The listing builds one solid part. Answer for the finished solid, in the listing's coordinates (mm). Round coordinates to 2 decimals unless told otherwise and drop trailing zeros. Loops run counter-clockwise (first coordinate to the right, second up) from the corner with the lowest first, then second, coordinate; pieces in that order, holes last. Notation, with made-up numbers: (-26.75, -37) -> (10.25, -37) arc R29 ccw to (10.25, -10) -> close; hole circle Ø7 at (72, 58). An arc over 180 degrees is marked (long way). Answer in a Markdown table with one row per item. Add a question column.
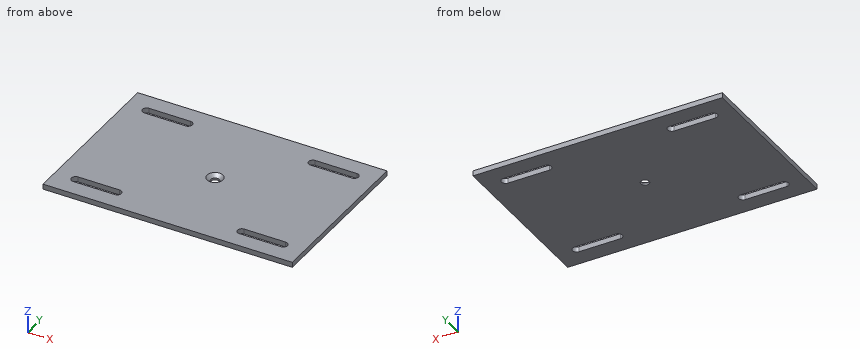
```python
from build123d import *

# Parameters (mm, degrees)
SKETCH1_W            = 152.4
SKETCH1_H            = 101.6
BOSS_EXTRUDE1_DEPTH  = 3.175
CUT_EXTRUDE1_DEPTH   = 92.636022529
MIRROR2_COPY_1_DEPTH = 92.636022529


with BuildPart() as part:
    # Sketch1 → Boss-Extrude1 (new body)
    with BuildSketch(Plane.XY):
        Rectangle(SKETCH1_W, SKETCH1_H)
    extrude(amount=BOSS_EXTRUDE1_DEPTH)

    # Sketch2 → Cut-Extrude1 (cut, symmetric)
    with BuildSketch(Plane.XY.offset(3.175)):
        with BuildLine():
            Line((-63.5, 40.665937046), (-38.1, 40.665937046))
            ThreePointArc((-38.1, 40.665937046), (-35.534062954, 38.1), (-38.1, 35.534062954))
            Line((-38.1, 35.534062954), (-63.5, 35.534062954))
            ThreePointArc((-63.5, 35.534062954), (-66.065937046, 38.1), (-63.5, 40.665937046))
        make_face()
    cut_extrude1 = extrude(amount=CUT_EXTRUDE1_DEPTH, both=True, mode=Mode.SUBTRACT)

    # Mirror1: Cut-Extrude1 across plane
    add(cut_extrude1.mirror(Plane(origin=(0, 0, 0), x_dir=(0, 0, 1), z_dir=(1, 0, 0))), mode=Mode.SUBTRACT)

    # Mirror2: Cut-Extrude1 across plane
    add(cut_extrude1.mirror(Plane.ZX), mode=Mode.SUBTRACT)

    # Mirror2 copy 1 sketch → Mirror2 copy 1 (cut, symmetric)
    with BuildSketch(Plane(origin=(0, 0, 3.175), x_dir=(-1, 0, 0), z_dir=(0, 0, 1))):
        with BuildLine():
            Line((-63.5, 40.665937046), (-38.1, 40.665937046))
            ThreePointArc((-38.1, 40.665937046), (-35.534062954, 38.1), (-38.1, 35.534062954))
            Line((-38.1, 35.534062954), (-63.5, 35.534062954))
            ThreePointArc((-63.5, 35.534062954), (-66.065937046, 38.1), (-63.5, 40.665937046))
        make_face()
    extrude(amount=MIRROR2_COPY_1_DEPTH, both=True, mode=Mode.SUBTRACT)

    # Sketch5 → CSK for #10 Flat Head Machine Screw (100)1 (revolve, cut)
    with BuildSketch(Plane(origin=(0, 0, 3.175), x_dir=(0, -1, 0), z_dir=(1, 0, 0))):
        Polygon((0, 0), (0, 3.175), (2.5527, 3.175), (2.5527, 1.960808018), (4.8895, 0), align=None)
    revolve(axis=Axis((0, 0, 9.525), (0, 0, -1)), mode=Mode.SUBTRACT)


solid = part.part
```
Item 1: Section C-C, the plane z = 0.5 is taken. Write down the section's boundary in (x, y).
Item 2: Flat-ended cylindrical pins translate along their axes: P1, Ø4, axis at x = 0, y = 0, coming from the +Z side; P2, Ø5, axis at x = 0, y = 27, coming from the -Z side. Find the tip coordinate at first contact, or state that the pin passes through.
Item 3: Section B-B, the plane y = 38.1 is taken. Write down the section's boundary in (x, z) (3 decimals).
Item 4: Consider L1, parallel to Y at x = -59.5, z = 2.9; L2, parallel to Y at x = 0, z = 0.9; L3, parallel to X at y = 0, z = 1.05. Determine where each line is inside the solid, lowest interval first. Write a range as from..to.
Item 5: Section A-A, the plane x = 42.5 is taken. Write down the section's boundary in (y, z) (3 decimals).
Here are the results:
| question | item | result |
|---|---|---|
| 1 | outline | (-76.2, -50.8) -> (76.2, -50.8) -> (76.2, 50.8) -> (-76.2, 50.8) -> close; hole (-63.5, -40.67) -> (-38.1, -40.67) arc R2.57 ccw to (-38.1, -35.53) -> (-63.5, -35.53) arc R2.57 ccw to start; hole (-63.5, 35.53) -> (-38.1, 35.53) arc R2.57 ccw to (-38.1, 40.67) -> (-63.5, 40.67) arc R2.57 ccw to start; hole circle Ø5.11 at (0, 0); hole (38.1, -40.67) -> (63.5, -40.67) arc R2.57 ccw to (63.5, -35.53) -> (38.1, -35.53) arc R2.57 ccw to start; hole (38.1, 35.53) -> (63.5, 35.53) arc R2.57 ccw to (63.5, 40.67) -> (38.1, 40.67) arc R2.57 ccw to start |
| 2 | P1 | passes through |
| 2 | P2 | stops at z = 0 |
| 3 | outline | (-76.2, 0) -> (-66.066, 0) -> (-66.066, 3.175) -> (-76.2, 3.175) -> close; (-35.534, 0) -> (35.534, 0) -> (35.534, 3.175) -> (-35.534, 3.175) -> close; (66.066, 0) -> (76.2, 0) -> (76.2, 3.175) -> (66.066, 3.175) -> close |
| 4 | L1 | y = -50.8..-40.67, -35.53..35.53, 40.67..50.8 |
| 4 | L2 | y = -50.8..-2.55, 2.55..50.8 |
| 4 | L3 | x = -76.2..-2.55, 2.55..76.2 |
| 5 | outline | (-50.8, 0) -> (-40.666, 0) -> (-40.666, 3.175) -> (-50.8, 3.175) -> close; (-35.534, 0) -> (35.534, 0) -> (35.534, 3.175) -> (-35.534, 3.175) -> close; (40.666, 0) -> (50.8, 0) -> (50.8, 3.175) -> (40.666, 3.175) -> close |
